from build123d import *

# Parameters (mm, degrees)
SKETCH006_R   = 3
SKETCH006_R_2 = 5.1
PAD003_DEPTH  = 40
POCKET_DEPTH  = 4.5
FILLET_R      = 1


with BuildPart() as part:
    # Sketch006 → Pad003 (new body)
    with BuildSketch(Plane.XZ.offset(-12.5)):
        with BuildLine():
            ThreePointArc((30.081867, 41.000372), (38.868733, 51.531528), (27.05887, 58.505866))
            ThreePointArc((25.786195, 58.494289), (26.423478, 58.396141), (27.05887, 58.505866))
            ThreePointArc((25.786195, 58.494289), (24.370225, 58.831452), (22.918423, 58.935953))
            Line((-97.076613, 57.844394), (22.918423, 58.935953))
            ThreePointArc((-97.076613, 57.844394), (-100.049297, 54.831898), (-97.051373, 51.844519))
            Line((-97.051373, 51.844519), (-3.880643, 51.780882))
            ThreePointArc((0.997022, 47.864886), (-0.75383, 50.679815), (-3.880643, 51.780882))
            ThreePointArc((0.997022, 47.864886), (4.182938, 42.770547), (9.864832, 40.816464))
            Line((30.081867, 41.000372), (9.864832, 40.816464))
        make_face()
        with Locations((30, 50)):
            Circle(SKETCH006_R, mode=Mode.SUBTRACT)
        with Locations((12.000745, 49.836266)):
            Circle(SKETCH006_R_2, mode=Mode.SUBTRACT)
    extrude(amount=PAD003_DEPTH)

    # Sketch007 → Pocket (cut, symmetric)
    with BuildSketch(Plane.XZ):
        with BuildLine():
            Line((-3.770677, 39.692385), (42.090467, 40.10957))
            Line((42.090467, 40.10957), (41.963118, 54.10899))
            Line((41.963118, 54.10899), (-1.987102, 53.709188))
            ThreePointArc((-1.987102, 53.709188), (-3.333238, 53.1372), (-3.880643, 51.780882))
            Line((-3.770677, 39.692385), (-3.880643, 51.780882))
        make_face()
    extrude(amount=POCKET_DEPTH, both=True, mode=Mode.SUBTRACT)

    # Fillet
    fillet_edges = [part.edges().sort_by_distance(p)[0] for p in [
        (38.025539, 0, 54.073171),
    ]]
    fillet(fillet_edges, radius=FILLET_R)


solid = part.part
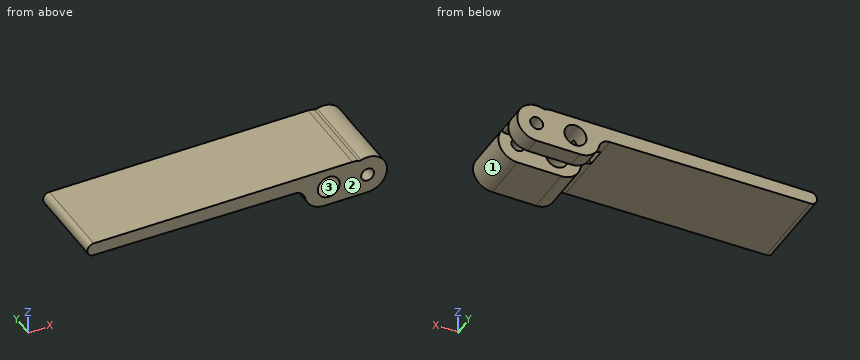
CAD build for the part. Positions are in the model's coordinates, mm. Face numbers are marked on the shaded views. Round coordinates to 2 decimals unless told otherwise and drop trailing zeros. Write each loop counter-clockwise with the first axis right and the second up, starting at its lowest first coordinate (ties: lowest second). Pieces come first, ordered by that corner, then holes.
(1) Mould opens along Z. For the marked faces 1, 2 and 3 say: pulls with the +Z half, pulls with the -Z half, needs draft (parallel to the pull), parting line crosses it, or undercut.
(2) Slice it at C-C, the plane y = 1. Write the cut outline in (x, z).
(3) Slice it at B-B, the plane y = 9. Write the cut outline in (x, z).
(4) Drop flat-ended pins along their axis: P1, Ø5, axis at x = 30, z = 50, coming from the +Y side; P2, Ø3, axis at y = -15, z = 53, coming from the -X side; P3, Ø10, axis at x = 24, y = -15.5, coming from the +Z side; P4, Ø6, axis at y = -8.5, z = 56, coming from the +X side. Give the stop position or say it passes through.
(5) Probe line 1 along Z through (x, y) = (30, 7.5); line 2 along Y through (x, z) = (28.5, 44.5); line 3 along X through (y, z) = (8.5, 51.25). List the from-to ranges inside material, lowest first.
(6) Slice it at D-D, the plane x = -10. Write the cut outline in (y, z).
(7) Slice it at A-A, the plane z = 42.25. Write the cut outline in (x, y), and give its area (3 significant figures).
From the geometry:
1. face 1: parting line crosses it
1. face 2: needs draft
1. face 3: undercut
2. outline: (-97.08, 57.84) arc R3 ccw to (-97.05, 51.84) - (-3.88, 51.78) arc R1.91 cw to (-1.99, 53.71) - (8.8, 53.81) arc R5.1 cw to (15.13, 53.86) - (36.21, 54.06) arc R1 ccw to (36.97, 55.69) arc R9 ccw to (27.06, 58.51) arc R2 cw to (25.79, 58.49) arc R9 ccw to (22.92, 58.94) - close
3. outline: (-97.08, 57.84) arc R3 ccw to (-97.05, 51.84) - (-3.88, 51.78) arc R5 cw to (1, 47.86) arc R9 ccw to (9.86, 40.82) - (30.08, 41) arc R9 ccw (long way) to (27.06, 58.51) arc R2 cw to (25.79, 58.49) arc R9 ccw to (22.92, 58.94) - close; hole circle Ø10.2 at (12, 49.84); hole circle Ø6 at (30, 50)
4. P1: passes through
4. P2: stops at x = -100.03
4. P3: stops at z = 58.94
4. P4: stops at x = 38.49
5. line 1: z = 41 to 47, 53 to 59
5. line 2: y = -27.5 to -4.5, 4.5 to 12.5
5. line 3: x = -1.64 to 7.1, 16.9 to 27.27, 32.73 to 38.91
6. outline: (-27.5, 51.79) - (12.5, 51.79) - (12.5, 58.64) - (-27.5, 58.64) - close
7. outline: (4.91, -27.5) - (34.58, -27.5) - (34.58, -4.5) - (4.91, -4.5) - close; (4.91, 4.5) - (34.58, 4.5) - (34.58, 12.5) - (4.91, 12.5) - close
7. area: 920 mm2
